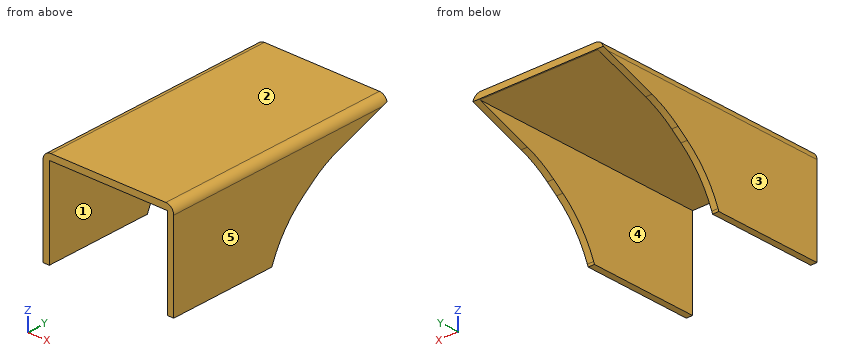
Solid Edge part; units mm, degrees
sketch "Sketch1" plane through (0, 0, 0) normal (0, 0, 1) x (1, 0, 0)
  line L0 (16.6, 30) -> (0, 30)
  line L1 (0, 30) -> (0, 0)
  line L2 (0, 0) -> (16.6, 0)
  line L3 (16.6, 0) -> (16.6, 30)
extrude "Protrusion1" add sketch "Sketch1" along normal blind 12
sketch "Sketch2" plane through (16.6, 15, 6) normal (1, 0, 0) x (0, 1, 0)
  line L0 (4.5259, 0.8255) -> (3.2238, -0.1545)
  arc A0 (-1.0985, -5.7305) -> (3.2238, -0.1545) centre (11.2888, -10.8694) cw
  line L1 (-1.0985, -5.7305) -> (-1.2103, -6)
  line L2 (-1.2103, -6) -> (15, -6)
  line L3 (15, -6) -> (15, 5.2385)
  line L4 (15, 5.2385) -> (8.1928, 2.8024)
  arc A1 (4.5259, 0.8255) -> (8.1928, 2.8024) centre (12.8653, -10.254) cw
extrude "ScavoEstrusione_1" cut sketch "Sketch2" against normal blind 87.395
sketch "Sketch3" plane through (8.3, 0, 6) normal (0, -1, 0) x (1, 0, 0)
  line L0 (7.5, 5.2) -> (7.5, -6)
  line L1 (-7.5, -6) -> (7.5, -6)
  line L2 (-7.5, -6) -> (-7.5, 5.2)
  line L3 (-7.5, 5.2) -> (7.5, 5.2)
extrude "ScavoEstrusione_2" cut sketch "Sketch3" against normal blind 100.7883
fillet "Rotondo_1" radius 1 2 edges at (0, 15, 12) (16.6, 15, 12)
The listing builds one solid part. Answer for the finished solid, in the listing's coordinates (mm). Face numbers are marked on the shaded views. A direction names the side the tool comes from. Round coordinates to 2 decimals unless told otherwise and drop trailing zeros. Write each loop counter-clockwise with the first axis right and the second up, starting at its lowest first coordinate (ties: lowest second). Pieces come first, ordered by that corner, then holes. Notation, with made-up numbers: (71.5, 17.5) - (75.5, 17.5) arc R23 cw to (75.5, 26.5) - close; hole circle Ø5 at (-21.5, -10.5). An arc over 180 degrees is marked (long way). Use a Markdown table: item, result. Add a question column.
1. The part is cut by section D-D (z = 7.75). Write down the section's boundary in (x, y), and give its area (3 significant figures).
2. A tool of negligible diameter and unlimited length cuts with its end or side. For the marked faces 1 and 2, from which of +Z, -Z, +X, -X, +Y, -Y can it reach the whole face along a straight path? Write none if from no direction.
3. For a pull along X with two mould halves and no side action, classify the marked faces 3, 4 and 5 as +X half, -X half, draft (parallel to the pull), parting line (faces both ways), or undercut.
4. The part is cut by section C-C (x = 7). Write down the section's boundary in (y, z).
5. Flat-ended cylindrical pins translate along their axes: P1, Ø4, axis at x = 7, y = 26.5, coming from the -Z side; P2, Ø1, axis at x = 3.5, z = 10, coming from the -Y side; P3, Ø6, axis at x = 3.5, z = 10.5, coming from the -Y side. Find the tip coordinate at first contact, or state that the pin passes through.
6. Consider line 1 (X direction, y = 5.5, z = 1.75); line 2 (Z direction, x = 15, y = 4.5); line 3 (Y direction, x = 16.25, z = 5.5). Determine where each line is inside the solid, lowest interval first.
7. The part is cut by section A-A (z = 1.5). Write down the section's boundary in (x, y).
8. The part is cut by section B-B (y = 9). Write down the section's boundary in (x, z), and give its area (3 significant figures).
Reported:
| question | item | result |
|---|---|---|
| 1 | outline | (0, 0) - (0.8, 0) - (0.8, 20.92) - (0, 20.92) - close; (15.8, 0) - (16.6, 0) - (16.6, 20.92) - (15.8, 20.92) - close |
| 1 | area | 33.5 mm^2 |
| 2 | face 1 | -Z, +Y, -Y |
| 2 | face 2 | +Z, +X, -X, +Y, -Y |
| 3 | face 3 | -X half |
| 3 | face 4 | undercut |
| 3 | face 5 | +X half |
| 4 | outline | (0, 11.2) - (29.89, 11.2) - (30, 11.24) - (30, 12) - (0, 12) - close |
| 5 | P1 | z = 11.2 |
| 5 | P2 | through |
| 5 | P3 | y = 0 |
| 6 | line 1 | 0 to 0.8, 15.8 to 16.6 |
| 6 | line 2 | 11.2 to 12 |
| 6 | line 3 | 0 to 17.78 |
| 7 | outline | (0, 0) - (0.8, 0) - (0.8, 14.49) - (0, 14.49) - close; (15.8, 0) - (16.6, 0) - (16.6, 14.49) - (15.8, 14.49) - close |
| 8 | outline | (0, 0) - (0.8, 0) - (0.8, 11.2) - (15.8, 11.2) - (15.8, 0) - (16.6, 0) - (16.6, 11) arc R1 ccw to (15.6, 12) - (1, 12) arc R1 ccw to (0, 11) - close |
| 8 | area | 30.8 mm^2 |
